Design review of the part built by this model. Coordinates are the model's own, in mm. Coordinates: 2 decimals unless noted, no trailing zeros. Write each loop counter-clockwise with the first axis right and the second up, starting at its lowest first coordinate (ties: lowest second). Pieces come first, ordered by that corner, then holes. Notation, with made-up numbers: (33.5, -4.5) -> (41.5, -4.5) arc R24 ccw to (41.5, 13.5) -> close; hole circle Ø3 at (61.25, 42.5). An arc over 180 degrees is marked (long way). Answer in a Markdown table with one row per item. Add a question column.
Item 1: To check wall thickness, follow line 1 (Y direction, x = -62, z = 0.95); line 2 (Y direction, x = 4, z = 0.25). State the ranges of each line that lie inside material, in increasing order.
Item 2: Take a section at C-C, the plane x = 0. Write out the cut boundary in (y, z), and give its area (3 significant figures).
Item 3: Take a section at B-B, the plane z = 0.45. Give the number of separate pieces and of enclosed holes in the cut face, and give its area (3 significant figures).
Item 4: Take a section at A-A, the plane x = -31. Write out the cut boundary in (y, z), and give its area (3 significant figures).
Item 5: Draft analysis for pull direction X (two halves, no side actions). For faces 1 (the face through (-2, 0, 0)), 2 (the face through (26.58, -9.63, 0.79)), state which applies: released by +X, released by -X, zero draft, split by the parting line, or undercut.
from build123d import *

# Parameters (mm, degrees)
SKETCH_W   = 217.93
SKETCH_H   = 52.58
SKETCH_R   = 6
SKETCH_R_2 = 4
SKETCH_R_3 = 1.6
SKETCH_R_4 = 9.5
SKETCH_R_5 = 5.25
SKETCH_W_2 = 12.65
SKETCH_H_2 = 11.5
PAD_DEPTH  = 1.6


with BuildPart() as part:
    # Sketch → Pad (new body)
    with BuildSketch(Plane.XY):
        Rectangle(SKETCH_W, SKETCH_H)
        with Locations((-93, -13.69)):
            Circle(SKETCH_R, mode=Mode.SUBTRACT)
        with Locations((-62, -13.69)):
            Circle(SKETCH_R, mode=Mode.SUBTRACT)
        with Locations((31, -13.69)):
            Circle(SKETCH_R, mode=Mode.SUBTRACT)
        with Locations((-31, -9.19)):
            Circle(SKETCH_R_2, mode=Mode.SUBTRACT)
        with Locations((-38.5, -9.19)):
            Circle(SKETCH_R_3, mode=Mode.SUBTRACT)
        with Locations((0, -11.69)):
            Circle(SKETCH_R_4, mode=Mode.SUBTRACT)
        with Locations((93, -15.19)):
            Circle(SKETCH_R_5, mode=Mode.SUBTRACT)
        with Locations((62, -16.19)):
            Rectangle(SKETCH_W_2, SKETCH_H_2, mode=Mode.SUBTRACT)
    extrude(amount=PAD_DEPTH)


solid = part.part
Answers:
| question | item | result |
|---|---|---|
| 1 | line 1 | y = -26.29 to -19.69, -7.69 to 26.29 |
| 1 | line 2 | y = -26.29 to -20.31, -3.07 to 26.29 |
| 2 | outline | (-26.29, 0) -> (-21.19, 0) -> (-21.19, 1.6) -> (-26.29, 1.6) -> close; (-2.19, 0) -> (26.29, 0) -> (26.29, 1.6) -> (-2.19, 1.6) -> close |
| 2 | area | 53.7 mm^2 |
| 3 | separate pieces | 1 |
| 3 | enclosed holes | 8 |
| 3 | area | 10,500 mm^2 |
| 4 | outline | (-26.29, 0) -> (-13.19, 0) -> (-13.19, 1.6) -> (-26.29, 1.6) -> close; (-5.19, 0) -> (26.29, 0) -> (26.29, 1.6) -> (-5.19, 1.6) -> close |
| 4 | area | 71.3 mm^2 |
| 5 | face 1 | zero draft |
| 5 | face 2 | undercut |
